```python
from build123d import *

# Parameters (mm, degrees)
SKETCH_6_W      = 80
SKETCH_6_H      = 40
SKETCH_6_W_2    = 76
SKETCH_6_H_2    = 36
SKETCH_14_W     = 40
SKETCH_14_H     = 80
EXTRUDE_1_DEPTH = 194
SKETCH_15_W     = 80
SKETCH_15_H     = 40
EXTRUDE_2_DEPTH = 595
EXTRUDE_3_DEPTH = 30
EXTRUDE_4_DEPTH = 30
EXTRUDE_5_DEPTH = 30


with BuildPart() as part:
    # По траектории13: sweep along a curve in space
    with BuildLine() as sweep_13_path:
        Line((0, 0, 0), (1000, 0, 0))
        Line((1000, 0, 0), (1000, -150, 0))
        Line((1000, -150, 0), (566.987298108, -400, 0))
        Line((566.987298108, -400, 0), (263.878406783, -225, 0))
        Line((263.878406783, -225, 0), (0, -147.584326952, 0))
        Line((0, -147.584326952, 0), (0, 0, 0))
    # Эскиз6 → По траектории13 (sweep)
    with BuildSketch(Plane(origin=(0, 0, 0), x_dir=(0, 0, -1), z_dir=(1, 0, 0))):
        with Locations((-0.551773823, -1.216505436)):
            Rectangle(SKETCH_6_W, SKETCH_6_H)
        with Locations((-0.551773823, -1.216505436)):
            Rectangle(SKETCH_6_W_2, SKETCH_6_H_2, mode=Mode.SUBTRACT)
    sweep(path=sweep_13_path.line, transition=Transition.RIGHT)

    # Эскиз14 → Бобышка-Вытянуть1 (add)
    with BuildSketch(Plane(origin=(-33.89376203, -115.529989888, 0), x_dir=(0.9595578428480989, -0.2815115383580276, 0), z_dir=(0.2815115383580276, 0.9595578428480989, 0))):
        with Locations((299.085913187, -0.551773823)):
            Rectangle(SKETCH_14_W, SKETCH_14_H)
    extrude(amount=EXTRUDE_1_DEPTH)

    # Эскиз15 → Бобышка-Вытянуть2 (add)
    with BuildSketch(Plane(origin=(306.181390541, -89.82636629, 0), x_dir=(0, 0, -1), z_dir=(0.9595578428480989, -0.28151153835802767, 0))):
        with Locations((-0.551773823, 51.50143726)):
            Rectangle(SKETCH_15_W, SKETCH_15_H)
    extrude(amount=EXTRUDE_2_DEPTH)

    # Эскиз17 → Бобышка-Вытянуть3 (add)
    with BuildSketch(Plane.XY.offset(40.551773823)):
        Polygon((-18.783494564, 18.783494564), (21.216505436, -21.216505436), (21.216505436, -131.698036755), (-18.783494564, -161.648850746), align=None)
    extrude(amount=EXTRUDE_3_DEPTH)

    # Эскиз18 → Бобышка-Вытянуть4 (add)
    with BuildSketch(Plane.XY.offset(40.551773823)):
        Polygon((272.28762851, -205.356356178), (256.433515773, -242.391001456), (566.987298108, -421.689311285), (566.987298108, -375.50128975), align=None)
    extrude(amount=EXTRUDE_4_DEPTH)

    # Эскиз19 → Бобышка-Вытянуть5 (add)
    with BuildSketch(Plane.XY.offset(40.551773823)):
        Polygon((1018.783494564, 18.783494564), (978.783494564, -21.216505436), (978.783494564, -137.750644875), (1018.783494564, -160.844655643), align=None)
    extrude(amount=EXTRUDE_5_DEPTH)


solid = part.part
```
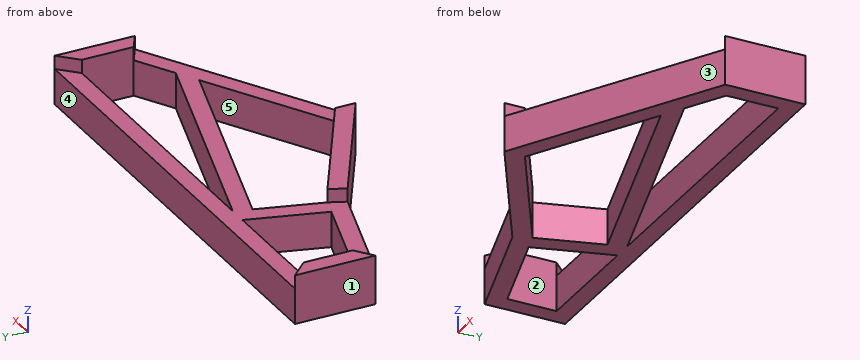
Geometry check sheet. Reference: the model listing, model coordinates, mm. Face numbers are marked on the shaded views. A direction names the side the tool comes from. Round coordinates to 2 decimals unless told otherwise and drop trailing zeros. Write each loop counter-clockwise with the first axis right and the second up, starting at its lowest first coordinate (ties: lowest second). Pieces come first, ordered by that corner, then holes. Notation, with made-up numbers: (-1.75, 45.25) - (44.25, 45.25) arc R24 ccw to (44.25, 68.25) - close; hole circle Ø11 at (5.25, 67). An arc over 180 degrees is marked (long way). Write each question's results on one line, items separated by ' | '.
(1) Set-up check for the marked faces 4 and 5: record each of +Z, -Z, +X, -X, +Y, -Y from which the full face is reachable in a straight line by a thin tool's end or side.
Computed:
face 4: +Z, -Z, +X, -X, +Y | face 5: +Z, -Z
(2) Draft check along Y on the marked faces 1, 2 and 3. Enter one of: pulls with the +Y half, pulls with the -Y half, needs draft (parallel to the pull), parting line crosses it, or undercut.
Computed:
face 1: needs draft | face 2: undercut | face 3: pulls with the -Y half
(3) Sectioned sample at A-A, the plane z = 53. Enter the section's corners in (x, y).
Computed:
outline: (-18.78, -161.65) - (21.22, -131.7) - (21.22, -21.22) - (-18.78, 18.78) - close; (256.43, -242.39) - (566.99, -421.69) - (566.99, -375.5) - (272.29, -205.36) - close; (978.78, -137.75) - (1018.78, -160.84) - (1018.78, 18.78) - (978.78, -21.22) - close
(4) Sectioned sample at C-C, the plane y = -315. Enter the section's corners in (x, z), plus the area to 3 significant figures.
Computed:
outline: (382.2, -39.45) - (462.2, -39.45) - (462.2, 70.55) - (382.2, 70.55) - close; (671.78, -39.45) - (751.78, -39.45) - (751.78, 40.55) - (671.78, 40.55) - close; hole (386.2, -37.45) - (458.2, -37.45) - (458.2, 38.55) - (386.2, 38.55) - close; hole (675.78, -37.45) - (747.78, -37.45) - (747.78, 38.55) - (675.78, 38.55) - close | area: 4,260 mm^2
(5) Sectioned sample at D-D, the plane x = 681. Enter the section's corners in (y, z), plus the area to 3 significant figures.
Computed:
outline: (-355.86, -39.45) - (-309.68, -39.45) - (-309.68, 40.55) - (-355.86, 40.55) - close; (-166.96, -39.45) - (-125.27, -39.45) - (-125.27, 40.55) - (-166.96, 40.55) - close; (-21.22, -39.45) - (18.78, -39.45) - (18.78, 40.55) - (-21.22, 40.55) - close; hole (-353.55, -37.45) - (-311.99, -37.45) - (-311.99, 38.55) - (-353.55, 38.55) - close; hole (-19.22, -37.45) - (16.78, -37.45) - (16.78, 38.55) - (-19.22, 38.55) - close | area: 4,330 mm^2
(6) Thickness scan on probe 1 along X at (y, z) = (-114, 46.5); probe 2 along Y at (x, z) = (861, -33); probe 3 along Y at (x, z) = (629, -0.5). Record the ranges inside material, lowest first. Write a range as from..to.
Computed:
probe 1: x = -18.78..21.22, 978.78..1018.78 | probe 2: y = -251.94..-249.63, -219.77..-178.08, -21.22..-19.22, 16.78..18.78 | probe 3: y = -385.89..-383.58, -342.01..-339.7, -151.7..-110.02, -21.22..-19.22, 16.78..18.78
(7) Sectioned sample at B-B, the plane x = 869. Enter the section's corners in (y, z), plus the area to 3 significant figures.
Computed:
outline: (-247.32, -39.45) - (-180.43, -39.45) - (-180.43, 40.55) - (-247.32, 40.55) - close; (-21.22, -39.45) - (18.78, -39.45) - (18.78, 40.55) - (-21.22, 40.55) - close; hole (-245.01, -37.45) - (-222.11, -37.45) - (-222.11, 38.55) - (-245.01, 38.55) - close; hole (-19.22, -37.45) - (16.78, -37.45) - (16.78, 38.55) - (-19.22, 38.55) - close | area: 4,080 mm^2
